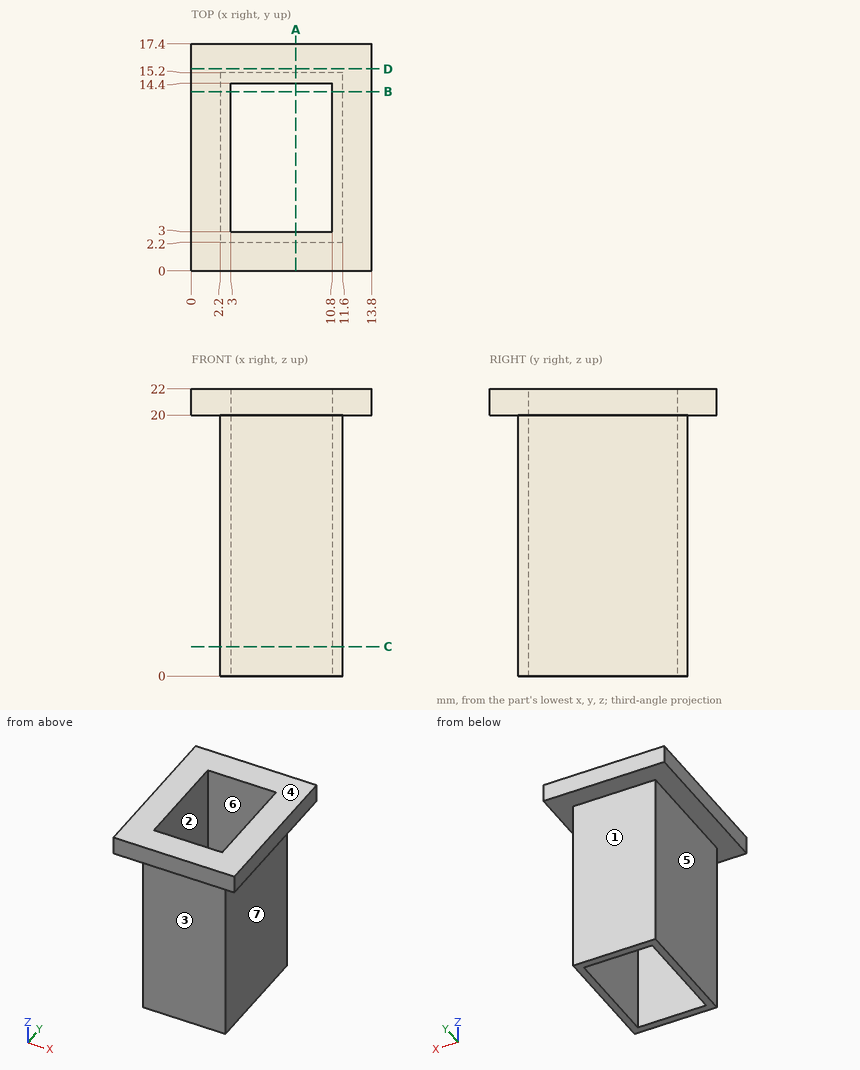
Here's the drawing with two shaded views (mm, measured from the low corner). I have some questions. A direction names the side the tool comes from. Coordinates: 2 decimals unless noted, no trailing zeros. Write each loop counter-clockwise with the first axis right and the second up, starting at its lowest first coordinate (ties: lowest second). Pieces come first, ordered by that corner, then holes. Notation, with made-up numbers: M 54,33.25 L 106,33.25 A24 ccw 106,44.25 Z; hole C 25,71.5 d7. An arc over 180 degrees is marked long. Answer as CSV lines item,"result".
Item 1: Imagine slicing it at C-C on z = 2.25. List the corners of the cut face in (x, y) for me.
Geometry results:
outline,"M 2.2,2.2 L 11.6,2.2 L 11.6,15.2 L 2.2,15.2 Z; hole M 3,3 L 10.8,3 L 10.8,14.4 L 3,14.4 Z"
Item 2: I'm going to push flat-ended pins straight in: P1, Ø8, axis at x = 9, y = 6.5, coming from the +Z side; P2, Ø6, axis at x = 8, z = 11, coming from the -Y side; P3, Ø3, axis at x = 4.5, z = 12.5, coming from the +Y side; P4, Ø1, axis at x = 9.5, y = 4.5, coming from the +Z side. Where does each tip first touch, or does it pass through?
Geometry results:
P1,"stops at z = 22"
P2,"stops at y = 2.2"
P3,"stops at y = 15.2"
P4,"passes through"
Item 3: Imagine slicing it at B-B on y = 13.75. List the corners of the cut face in (x, z) for me, plus the area to 3 significant figures.
Geometry results:
outline,"M 0,20 L 2.2,20 L 2.2,0 L 3,0 L 3,22 L 0,22 Z; M 10.8,0 L 11.6,0 L 11.6,20 L 13.8,20 L 13.8,22 L 10.8,22 Z"
area,"44.0 mm2"
Item 4: Imagine slicing it at D-D on y = 15.5. List the corners of the cut face in (x, z) for me, plus the area to 3 significant figures.
Geometry results:
outline,"M 0,20 L 13.8,20 L 13.8,22 L 0,22 Z"
area,"27.6 mm2"
Item 5: We'd pull the mould along X, two halves only. Please class the marked faces 4, 5, 6 and 7: +X half, -X half, draft (parallel to the pull), parting line (faces both ways), or undercut.
Geometry results:
face 4,"draft"
face 5,"-X half"
face 6,"undercut"
face 7,"+X half"
Item 6: On a 3-axis mill with a long thin cutter (end or side, diameter ignored), from which of +Z, -Z, +X, -X, +Y, -Y can I reach the whole of each face in a straight line? I mean the marked faces 1, 2 and 3. Say none if no direction works.
Geometry results:
face 1,"-Z, +X, -X, +Y"
face 2,"+Z, -Z"
face 3,"-Z, +X, -X, -Y"
Item 7: Imagine slicing it at A-A on x = 8. List the corners of the cut face in (y, z) for me.
Geometry results:
outline,"M 0,20 L 2.2,20 L 2.2,0 L 3,0 L 3,22 L 0,22 Z; M 14.4,0 L 15.2,0 L 15.2,20 L 17.4,20 L 17.4,22 L 14.4,22 Z"
Item 8: Please list where these lines run through material, in increasing order: line 1 along X through (y, z) = (11, 19); line 2 along Y through (x, z) = (7.25, 18.25); line 3 along X through (y, z) = (2.25, 8.5).
Geometry results:
line 1,"x = 2.2 to 3, 10.8 to 11.6"
line 2,"y = 2.2 to 3, 14.4 to 15.2"
line 3,"x = 2.2 to 11.6"
